Geometry check sheet. Reference: the model listing, model coordinates, mm. A direction names the side the tool comes from. Round coordinates to 2 decimals unless told otherwise and drop trailing zeros. Write each loop counter-clockwise with the first axis right and the second up, starting at its lowest first coordinate (ties: lowest second). Pieces come first, ordered by that corner, then holes. Notation, with made-up numbers: M 85.5,10.5 L 105.5,10.5 A21 cw 105.5,19.5 Z; hole C -11.75,66.25 d10. An arc over 180 degrees is marked long. Put each result on its own line as item: value. Start each with the question number.
(1) Material ranges on probe 1 along Z at (x, y) = (0, -20.9); probe 2 along Y at (x, z) = (-1.5, 27) (3 decimals); probe 3 along Z at (x, y) = (7.5, -12) (3 decimals), recorded low to high.
(2) Section check A-A on x = 0. Record the cut outline in (y, z) (3 decimals).
(3) Gauge pin test, flat end, axial feed: pin 1 (1 mm diameter, centred on x = -6, y = -16.5, fed in from +Z) (3 decimals). Record the tip position at first contact, or that the pin passes through.
(4) Mould release check, pull along X, two halves, no side actions. Record for faces 1 (the cylindrical face through (0.73, -20.62, 15.75)), 2 (the flat face through (0, 19.05, 14)), 3 (the flat face through (12.7, 2, 3)): pulls with the +X half, pulls with the -X half, needs draft (parallel to the pull), parting line crosses it, or undercut.
(5) Section check D-D on x = 4.75. Record the cut outline in (y, z) (3 decimals).
(6) Section check C-C on z = 29.5. Record the cut outline in (x, y) (3 decimals), then the cut area to 3 significant figures.
(7) Tool access check on faces 4 (the flat face through (-3, -22.225, 16)), 5 (the flat face through (0, 0, 3.175)). Record the directions out of +Z, -Z, +X, -X, +Y, -Y that give a thin tool (end or side, any length) a straight path to the whole face; none if there is none.
(8) Section check B-B on z = 19.05. Record the cut outline in (x, y) (3 decimals).
from build123d import *

# Parameters (mm, degrees)
F1_DEPTH = 12.7
F3_D     = 6.7564


with BuildPart() as f1:
    # F0 (on Right) → F1 (new body, symmetric)
    with BuildSketch(Plane.YZ):
        Polygon((-22.225, 31.75), (-22.225, 0), (0, 0), (0, 3.175), (-19.05, 3.175), (-19.05, 31.75), align=None)
        Polygon((0, 3.175), (0, 0), (22.225, 0), (22.225, 31.75), (19.05, 31.75), (19.05, 3.175), align=None)
    extrude(amount=F1_DEPTH, both=True)

    # F3 (through all)
    with Locations(Plane.XZ.offset(22.225)):
        with Locations((0, 19.05)):
            Hole(F3_D / 2)


solid = f1.part
Answers follow:
1. probe 1: z = 0 to 15.67, 22.43 to 31.75
1. probe 2: y = -22.225 to -19.05, 19.05 to 22.225
1. probe 3: z = 0 to 3.175
2. outline: M -22.225,0 L 22.225,0 L 22.225,15.672 L 19.05,15.672 L 19.05,3.175 L -19.05,3.175 L -19.05,15.672 L -22.225,15.672 Z; M -22.225,22.428 L -19.05,22.428 L -19.05,31.75 L -22.225,31.75 Z; M 19.05,22.428 L 22.225,22.428 L 22.225,31.75 L 19.05,31.75 Z
3. pin 1: stops at z = 3.175
4. face 1: undercut
4. face 2: needs draft
4. face 3: pulls with the +X half
5. outline: M -22.225,0 L 22.225,0 L 22.225,31.75 L 19.05,31.75 L 19.05,3.175 L -19.05,3.175 L -19.05,31.75 L -22.225,31.75 Z
6. outline: M -12.7,-22.225 L 12.7,-22.225 L 12.7,-19.05 L -12.7,-19.05 Z; M -12.7,19.05 L 12.7,19.05 L 12.7,22.225 L -12.7,22.225 Z
6. area: 161 mm^2
7. face 4: +Z, -Z, +X, -X, -Y
7. face 5: +Z, +X, -X
8. outline: M -12.7,-22.225 L -3.378,-22.225 L -3.378,-19.05 L -12.7,-19.05 Z; M -12.7,19.05 L -3.378,19.05 L -3.378,22.225 L -12.7,22.225 Z; M 3.378,-22.225 L 12.7,-22.225 L 12.7,-19.05 L 3.378,-19.05 Z; M 3.378,19.05 L 12.7,19.05 L 12.7,22.225 L 3.378,22.225 Z
